Model file for the job. Use its own axes, mm. A direction names the side the tool comes from. Give positions to 0.01 mm unless a question says otherwise; leave off trailing zeros. Write each loop counter-clockwise with the first axis right and the second up, starting at its lowest first coordinate (ties: lowest second). Pieces come first, ordered by that corner, then holes. Notation, with made-up numbers: (49.25, -38.5) - (56.25, -38.5) arc R32 ccw to (56.25, -12.5) - close; hole circle Ø1 at (-29.5, 12.25). An arc over 180 degrees is marked (long way). One line per item, written item: value. Start each with the question number.
(1) Cut at C-C, the plane z = 6. List the corners of the cut face in (x, y).
(2) Cut at D-D, the plane x = 11. List the corners of the cut face in (y, z).
(3) Cut at B-B, the plane x = -5. State how many separate pieces and enclosed holes the cut face has, and give its area (3 significant figures).
(4) Cut at A-A, the plane y = -17.5. List the corners of the cut face in (x, z), and give its area (3 significant figures).
(5) 3-axis set-ups, long thin cutter, end or side, ignore diameter. For faces 1 (the face through (13.2, -13.2, 2.6)), 2 (the face through (1, -18, 0)), 3 (the face through (-10.2, -21, 20.1)): which of +Z, -Z, +X, -X, +Y, -Y reach the whole face in a straight line?
(6) Mould opens along X. For faces 4 (the face through (-5.133, -13.169, 1.095)), 5 (the face through (4, -11, 15)), 6 (the face through (-9.868, -23.535, 26.349)), 7 (the face through (-14, -19, 20)) say: pulls with the +X half, pulls with the -X half, needs draft (parallel to the pull), parting line crosses it, or undercut.
(7) Probe L1, parallel to Z at x = 10, y = -12.4; L2, parallel to Z at x = 10, y = -19.75; L3, parallel to Z at x = -6, y = -12.65. List the from-to ranges inside material, lowest first.
(8) Drop flat-ended pins along their axis: P1, Ø1.5, axis at x = -10.5, y = -13.5, coming from the -Z side; P2, Ø4, axis at x = -4.5, z = 35, coming from the +Y side; P3, Ø11.5, axis at x = -5, z = 20, coming from the -Y side; P4, Ø6.5, axis at x = 11.5, z = 35, coming from the +Y side. Give the stop position or say it passes through.
from build123d import *

# Parameters (mm, degrees)
EXTRUDE_1_DEPTH             = 40
SKETCH_9_R                  = 5
CUT_EXTRUDE_3_DEPTH         = 52.078371156
SKETCH_16_OUTSIDE_W         = 42.358
SKETCH_16_OUTSIDE_H         = 53.358
SKETCH_16_OUTSIDE_R         = 9
CUT_EXTRUDE_4_DEPTH         = 13
HOLE_WIZARD_M41_D           = 4.5
HOLE_WIZARD_M41_CBORE_D     = 8
HOLE_WIZARD_M41_CBORE_DEPTH = 4.4
SKETCH_19_R                 = 8
CUT_EXTRUDE_5_DEPTH         = 5


with BuildPart() as part:
    # Эскиз1 → Бобышка-Вытянуть1 (new body)
    with BuildSketch(Plane.XY):
        Polygon((7.5, 0), (7.5, -11), (15, -11), (15, -26), (-14, -26), (-14, 2), (0, 2), (7.5, 2), align=None)
    extrude(amount=EXTRUDE_1_DEPTH)

    # Эскиз9 → Вырез-Вытянуть3 (cut, through all)
    with BuildSketch(Plane(origin=(0, 2, 0), x_dir=(1, 0, 0), z_dir=(0, 1, 0))):
        with Locations(Location((-5, -20, 0), (0, 0, 180))):
            Circle(SKETCH_9_R)
    extrude(amount=-CUT_EXTRUDE_3_DEPTH, mode=Mode.SUBTRACT)

    # Эскиз16 outside → Вырез-Вытянуть4 (cut)
    with BuildSketch(Plane(origin=(0, 2, 0), x_dir=(1, 0, 0), z_dir=(0, 1, 0))):
        with Locations((0.5, -20)):
            Rectangle(SKETCH_16_OUTSIDE_W, SKETCH_16_OUTSIDE_H)
        with Locations(Location((-5, -20, 0), (0, 0, 180))):
            Circle(SKETCH_16_OUTSIDE_R, mode=Mode.SUBTRACT)
    extrude(amount=-CUT_EXTRUDE_4_DEPTH, mode=Mode.SUBTRACT)

    # Цековка для  винта с внутренним шестигранником M41 (through all)
    with Locations(Plane(origin=(0, -11, 0), x_dir=(-1, 0, 0), z_dir=(0, 1, 0))):
        with Locations((-10, 35), (-10, 5), (6, 35), (6, 5)):
            CounterBoreHole(HOLE_WIZARD_M41_D / 2, HOLE_WIZARD_M41_CBORE_D / 2, HOLE_WIZARD_M41_CBORE_DEPTH)

    # Эскиз19 → Вырез-Вытянуть5 (cut)
    with BuildSketch(Plane.XZ.offset(26)):
        with Locations(Location((-5, 20, 0), (0, 0, 270))):
            Circle(SKETCH_19_R)
    extrude(amount=-CUT_EXTRUDE_5_DEPTH, mode=Mode.SUBTRACT)


solid = part.part
Answers follow:
1. outline: (-14, -26) - (-8.02, -26) - (-8.02, -15.4) - (-9.87, -15.4) - (-9.87, -11) - (-14, -11) - close; (-3.98, -26) - (7.98, -26) - (7.98, -15.4) - (6.13, -15.4) - (6.13, -11) - (-2.13, -11) - (-2.13, -15.4) - (-3.98, -15.4) - close; (12.02, -26) - (15, -26) - (15, -11) - (13.87, -11) - (13.87, -15.4) - (12.02, -15.4) - close
2. outline: (-26, 0) - (-11, 0) - (-11, 1.13) - (-15.4, 1.13) - (-15.4, 2.98) - (-26, 2.98) - close; (-26, 7.02) - (-15.4, 7.02) - (-15.4, 8.87) - (-11, 8.87) - (-11, 31.13) - (-15.4, 31.13) - (-15.4, 32.98) - (-26, 32.98) - close; (-26, 37.02) - (-15.4, 37.02) - (-15.4, 38.87) - (-11, 38.87) - (-11, 40) - (-26, 40) - close
3. separate pieces: 4
3. enclosed holes: 0
3. area: 370 mm²
4. outline: (-14, 0) - (15, 0) - (15, 40) - (-14, 40) - close; hole circle Ø10 at (-5, 20); hole circle Ø4.5 at (-6, 5); hole circle Ø4.5 at (-6, 35); hole circle Ø4.5 at (10, 5); hole circle Ø4.5 at (10, 35)
4. area: 1,020 mm²
5. face 1: +Y
5. face 2: -Z, +X, -X, +Y, -Y
5. face 3: -Y
6. face 4: undercut
6. face 5: needs draft
6. face 6: undercut
6. face 7: pulls with the -X half
7. L1: z = 0 to 1, 9 to 31, 39 to 40
7. L2: z = 0 to 2.75, 7.25 to 32.75, 37.25 to 40
7. L3: z = 0 to 1, 9 to 15.1, 24.9 to 31, 39 to 40
8. P1: stops at z = 0
8. P2: stops at y = -15.4
8. P3: stops at y = -21
8. P4: stops at y = -11
